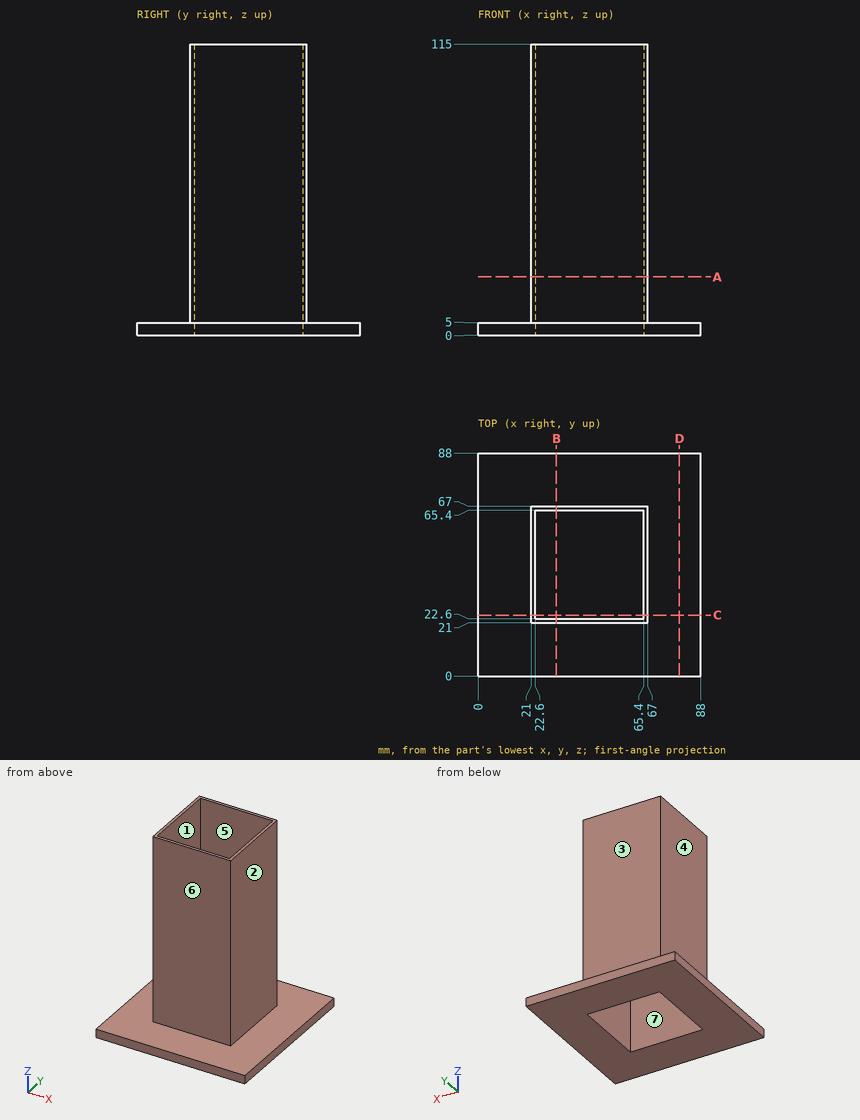
The figure shows three views and two pictorial views of one solid part (mm, origin at its lowest corner). Answer the questions. A direction names the side the tool comes from. Give positions to 0.01 mm unless a question says otherwise; leave off trailing zeros. Order: outer loops, then holes, each group sorted by start corner. A loop starts at its lowest first (then second) coordinate and runs counter-clockwise, first axis right, second up. Notation, with made-up numbers: M 55,-13.75 L 70,-13.75 A25 ccw 70,-0.75 Z; hole C -40,-5 d6. An arc over 180 degrees is marked long. Return JSON: item names as keys, results as strings.
1) Section D-D, the plane x = 79.5 is taken. Write down the section's boundary in (y, z), plus the area to 3 significant figures.
Resolved:
{"outline": "M 0,0 L 88,0 L 88,5 L 0,5 Z", "area": "440 mm^2"}
2) Section A-A, the plane z = 23 is taken. Write down the section's boundary in (x, y).
Resolved:
{"outline": "M 21,21 L 67,21 L 67,67 L 21,67 Z; hole M 22.6,22.6 L 65.4,22.6 L 65.4,65.4 L 22.6,65.4 Z"}
3) Straight lines are drawn through the part: line 1 along Y through (x, z) = (30.5, 79); line 2 along Z through (x, y) = (12, 68). For each, find the intervals that lie inside material, in ascending order. Write a range as [from, to].
Resolved:
{"line 1": "[21, 22.6], [65.4, 67]", "line 2": "[0, 5]"}
4) Each of these flat-tipped pins is pushed along its axis until it touches: pin 1 (1 mm diameter, centred on y = 24.5, z = 24, fed in from -X); pin 2 (21.5 mm diameter, centred on y = 51.5, z = 78.5, fed in from +X); pin 3 (21.5 mm diameter, centred on x = 44.5, z = 47, fed in from -Y). Where does it stop, or does it pass through?
Resolved:
{"pin 1": "x = 21", "pin 2": "x = 67", "pin 3": "y = 21"}
5) For a pull along X with two mould halves and no side action, classify the marked faces 4, 5, 6 and 7 as +X half, -X half, draft (parallel to the pull), parting line (faces both ways), or undercut.
Resolved:
{"face 4": "-X half", "face 5": "undercut", "face 6": "draft", "face 7": "undercut"}
6) Section B-B, the plane x = 31 is taken. Write down the section's boundary in (y, z), plus the area to 3 significant figures.
Resolved:
{"outline": "M 0,0 L 22.6,0 L 22.6,115 L 21,115 L 21,5 L 0,5 Z; M 65.4,0 L 88,0 L 88,5 L 67,5 L 67,115 L 65.4,115 Z", "area": "578 mm^2"}
7) A tool of negligible diameter and unlimited length cuts with its end or side. For the marked faces 1, 2 and 3, from which of +Z, -Z, +X, -X, +Y, -Y can it reach the whole face along a straight path? Write none if from no direction.
Resolved:
{"face 1": "+Z, -Z", "face 2": "+Z, +X, +Y, -Y", "face 3": "+Z, +X, -X, +Y"}
